Read the model definition and answer for the solid it produces. Units are mm, in the model's axes. Round coordinates to 2 decimals unless told otherwise and drop trailing zeros. Order: outer loops, then holes, each group sorted by start corner. A loop starts at its lowest first (then second) coordinate and runs counter-clockwise, first axis right, second up. Notation, with made-up numbers: (62.5, 5) -> (111.5, 5) arc R24 ccw to (111.5, 28) -> close; hole circle Ø6 at (44, -17.5). An arc over 180 degrees is marked (long way). Use a Markdown table: item, result. Add a question column.
1. Section A-A, the plane y = -0.25 is taken. Give the vertices of the cut face in (x, z), then the cut area to 3 significant figures.
2. Section B-B, the plane x = -6 is taken. Give the vertices of the cut face in (y, z).
3. Given pin 1 (4 mm diameter, centred on x = -5, y = 8.5, fed in from +Z); pin 2 (1.5 mm diameter, centred on y = 7, z = 2.5, fed in from -X); pin 3 (1 mm diameter, centred on y = 5, z = 2.5, fed in from -X), each flat-ended and moving along its own axis, determine where each tip first touches the part or whether it passes through.
4. Consider L1, parallel to Y at x = -0.25, z = 0.7; L2, parallel to X at y = -4.5, z = 2.1; L3, parallel to X at y = -3.5, z = 2.75. Determine where each line is inside the solid, lowest interval first. Write a range as [from, to].
5. Section C-C, the plane z = 1.7 is taken. Give the vertices of the cut face in (x, y).
6. The mould has two halves that part along X. Classify faces 1 (the face through (-4.93, 3.01, 1.48)), 2 (the face through (0.81, 8.19, 1.48)), 3 (the face through (0, 3, 0)): +X half, -X half, draft (parallel to the pull), parting line (faces both ways), or undercut.
7. Section D-D, the plane y = -4.5 is taken. Give the vertices of the cut face in (x, z), then the cut area to 3 significant figures.
```python
from build123d import *

# Parameters (mm, degrees)
SKETCH_1_R      = 1.5
SKETCH_1_R_2    = 2.75
EXTRUDE_1_DEPTH = 3


with BuildPart() as part:
    # 草图1 → 凸台-拉伸1 (new body)
    with BuildSketch(Plane.XY):
        Polygon((0, 11.547005384), (-10, -5.773502692), (10, -5.773502692), align=None)
        with Locations((0, 6.92820323)):
            Circle(SKETCH_1_R, mode=Mode.SUBTRACT)
        with Locations((-6, -3.464101615)):
            Circle(SKETCH_1_R, mode=Mode.SUBTRACT)
        with Locations((6, -3.464101615)):
            Circle(SKETCH_1_R, mode=Mode.SUBTRACT)
        Circle(SKETCH_1_R_2, mode=Mode.SUBTRACT)
    extrude(amount=EXTRUDE_1_DEPTH)


solid = part.part
```
Verdict:
| question | item | result |
|---|---|---|
| 1 | outline | (-6.81, 0) -> (-2.74, 0) -> (-2.74, 3) -> (-6.81, 3) -> close; (2.74, 0) -> (6.81, 0) -> (6.81, 3) -> (2.74, 3) -> close |
| 1 | area | 24.4 mm2 |
| 2 | outline | (-5.77, 0) -> (-4.96, 0) -> (-4.96, 3) -> (-5.77, 3) -> close; (-1.96, 0) -> (1.15, 0) -> (1.15, 3) -> (-1.96, 3) -> close |
| 3 | pin 1 | passes through |
| 3 | pin 2 | stops at x = -3.06 |
| 3 | pin 3 | stops at x = -4.07 |
| 4 | L1 | y = [-5.77, -2.74], [2.74, 5.45], [8.41, 11.11] |
| 4 | L2 | x = [-9.26, -7.08], [-4.92, 4.92], [7.08, 9.26] |
| 4 | L3 | x = [-8.69, -7.5], [-4.5, 4.5], [7.5, 8.69] |
| 5 | outline | (-10, -5.77) -> (10, -5.77) -> (0, 11.55) -> close; hole circle Ø3 at (-6, -3.46); hole circle Ø5.5 at (0, 0); hole circle Ø3 at (0, 6.93); hole circle Ø3 at (6, -3.46) |
| 6 | face 1 | -X half |
| 6 | face 2 | undercut |
| 6 | face 3 | draft |
| 7 | outline | (-9.26, 0) -> (-7.08, 0) -> (-7.08, 3) -> (-9.26, 3) -> close; (-4.92, 0) -> (4.92, 0) -> (4.92, 3) -> (-4.92, 3) -> close; (7.08, 0) -> (9.26, 0) -> (9.26, 3) -> (7.08, 3) -> close |
| 7 | area | 42.6 mm2 |
